Can you work these out from the model? Positions are in its coordinate system, mm. A direction names the side the tool comes from. Give positions to 0.01 mm unless a question says otherwise; leave off trailing zeros. Order: outer loops, then holes, each group sorted by start corner. A loop starts at its lowest first (then second) coordinate and runs counter-clockwise, first axis right, second up. Notation, with made-up numbers: M 52,-33 L 110,-33 A21 ccw 110,-21 Z; hole C 73.25,53.25 d8. An arc over 180 degrees is marked long. Answer as a JSON object with one key per item and string values.
```python
from build123d import *

# Parameters (mm, degrees)
SKETCH1_R           = 4
SKETCH1_R_2         = 1.5
BOSS_EXTRUDE1_DEPTH = 5
SKETCH2_W           = 8
SKETCH2_H           = 5
CUT_EXTRUDE1_DEPTH  = 10
SKETCH3_R           = 1.5
CUT_EXTRUDE2_DEPTH  = 10
CUT_EXTRUDE3_DEPTH  = 10


with BuildPart() as part:
    # Sketch1 → Boss-Extrude1 (new body)
    with BuildSketch(Plane.XY):
        with BuildLine():
            Line((-12.5, 0), (-12.5, -77.5))
            Line((-12.5, -77.5), (12.5, -77.5))
            Line((12.5, -77.5), (12.5, 0))
            ThreePointArc((12.5, 0), (0, 12.5), (-12.5, 0))
        make_face()
        Circle(SKETCH1_R, mode=Mode.SUBTRACT)
        with Locations((0, 7)):
            Circle(SKETCH1_R_2, mode=Mode.SUBTRACT)
        with Locations((4.949747468, 4.949747468)):
            Circle(SKETCH1_R_2, mode=Mode.SUBTRACT)
        with Locations((7, 0)):
            Circle(SKETCH1_R_2, mode=Mode.SUBTRACT)
        with Locations((4.949747468, -4.949747468)):
            Circle(SKETCH1_R_2, mode=Mode.SUBTRACT)
        with Locations((0, -7)):
            Circle(SKETCH1_R_2, mode=Mode.SUBTRACT)
        with Locations((-4.949747468, -4.949747468)):
            Circle(SKETCH1_R_2, mode=Mode.SUBTRACT)
        with Locations((-7, 0)):
            Circle(SKETCH1_R_2, mode=Mode.SUBTRACT)
        with Locations((-4.949747468, 4.949747468)):
            Circle(SKETCH1_R_2, mode=Mode.SUBTRACT)
    extrude(amount=BOSS_EXTRUDE1_DEPTH)

    # Sketch2 → Cut-Extrude1 (cut)
    with BuildSketch(Plane.XY.offset(5)):
        with Locations((0, -43)):
            Rectangle(SKETCH2_W, SKETCH2_H)
    extrude(amount=-CUT_EXTRUDE1_DEPTH, mode=Mode.SUBTRACT)

    # Sketch3 → Cut-Extrude2 (cut)
    with BuildSketch(Plane.XY.offset(5)):
        with Locations((0, -65)):
            Circle(SKETCH3_R)
        with Locations((0, -58)):
            Circle(SKETCH3_R)
        with Locations((-7, -65)):
            Circle(SKETCH3_R)
        with Locations((7, -65)):
            Circle(SKETCH3_R)
        with Locations((0, -72)):
            Circle(SKETCH3_R)
    extrude(amount=-CUT_EXTRUDE2_DEPTH, mode=Mode.SUBTRACT)

    # Sketch4 → Cut-Extrude3 (cut)
    with BuildSketch(Plane.XY.offset(5)):
        with BuildLine():
            Line((5, -20), (5, -28))
            Line((5, -28), (12.5, -35.5))
            Line((12.5, -35.5), (12.5, -27.5))
            ThreePointArc((12.5, -27.5), (17.803300859, -14.696699141), (5, -20))
        make_face()
    extrude(amount=-CUT_EXTRUDE3_DEPTH, mode=Mode.SUBTRACT)


solid = part.part
```
1) I want a section at A-A on y = -43. Write out the boundary of the cut face in (x, z), and give its area (3 significant figures).
Results found:
{"outline": "M -12.5,0 L -4,0 L -4,5 L -12.5,5 Z; M 4,0 L 12.5,0 L 12.5,5 L 4,5 Z", "area": "85.0 mm²"}
2) I'm going to push flat-ended pins straight in: pin 1 Ø2.5 at (x, y) = (0, -58) entering from -Z; pin 2 Ø2.5 at (x, z) = (-2, 2) entering from +Y. Where does each tip first touch, or does it pass through?
Results found:
{"pin 1": "passes through", "pin 2": "stops at y = 12.48"}
3) I need wall thicknesses on L1, parallel to X at y = -65, z = 3.3; L2, parallel to Y at x = -1.75, z = 2; L3, parallel to Y at x = -5, z = 4.75. Which ranges of each line are inside material? Lowest first, please.
Results found:
{"L1": "x = -12.5 to -8.5, -5.5 to -1.5, 1.5 to 5.5, 8.5 to 12.5", "L2": "y = -77.5 to -45.5, -40.5 to -3.6, 3.6 to 12.38", "L3": "y = -77.5 to -6.45, -3.45 to 3.45, 6.45 to 11.46"}
4) I want a section at B-B on x = 0. Count the separate pieces of the cut face and the enclosed holes in it, and give its area (3 significant figures).
Results found:
{"separate pieces": "8", "enclosed holes": "0", "area": "310 mm²"}
5) Thinking about a two-plate mould opening in Y: for faces 4 (the face through (9, -32, 3)), 5 (the face through (0.275, 12.497, 2.465)), 6 (the face through (12.5, -57, 2)), which applies, pulls with the +Y half, pulls with the -Y half, needs draft (parallel to the pull), parting line crosses it, or undercut?
Results found:
{"face 4": "undercut", "face 5": "pulls with the +Y half", "face 6": "needs draft"}
6) For faces 1 (the face through (0, -45.5, 3)), 2 (the face through (7.255, -14.639, 2.535)), 3 (the face through (0, -32, 5)), which set-ups out of +Z, -Z, +X, -X, +Y, -Y let a thin tool reach every point of the face, with its end or its side?
Results found:
{"face 1": "+Z, -Z", "face 2": "+Z, -Z, +X", "face 3": "+Z, +X, -X, +Y, -Y"}
7) I want a section at C-C on x = 10.5. Write out the boundary of the cut face in (y, z).
Results found:
{"outline": "M -77.5,0 L -33.5,0 L -33.5,5 L -77.5,5 Z; M -12.77,0 L 6.78,0 L 6.78,5 L -12.77,5 Z"}
